from build123d import *

# Parameters (mm, degrees)
ESQUISSE1_R                  = 65
BOSS_EXTRU_1_DEPTH           = 8
ESQUISSE2_R                  = 63
ENL_V_MAT_EXTRU_1_DEPTH      = 6
BOSS_EXTRU_2_DEPTH           = 6
R_P_TITION_CIRCULAIRE1_COUNT = 8
COQUE1_DEPTH                 = 8
CHAMFER1_SIZE                = 3


# Read off the part's stored shape, not the designer's step: Coque1
with BuildPart() as part:
    # Esquisse1 → Boss.-Extru.1 (new body)
    with BuildSketch(Plane(origin=(0, 0, 0), x_dir=(1, 0, 0), z_dir=(0, 1, 0))):
        with Locations(Location((0, 0, 0), (0, 0, 270))):
            Circle(ESQUISSE1_R)
    extrude(amount=BOSS_EXTRU_1_DEPTH)

    # Esquisse2 → Enlèv. mat.-Extru.1 (cut)
    with BuildSketch(Plane(origin=(0, 8, 0), x_dir=(1, 0, 0), z_dir=(0, 1, 0))):
        with Locations(Location((0, 0, 0), (0, 0, 270))):
            Circle(ESQUISSE2_R)
    extrude(amount=-ENL_V_MAT_EXTRU_1_DEPTH, mode=Mode.SUBTRACT)

    # Esquisse3 → Boss.-Extru.2 (add)
    with BuildSketch(Plane(origin=(0, 2, 0), x_dir=(1, 0, 0), z_dir=(0, 1, 0))):
        with BuildLine():
            Line((-41.321316613, -33.189588629), (-17.610927668, -9.479199685))
            ThreePointArc((-17.610927668, -9.479199685), (-18.47759065, -7.653668647), (-19.155612754, -5.75))
            Line((-19.155612754, -5.75), (-52.687166369, -5.75))
            ThreePointArc((-52.687166369, -5.75), (-48.965615223, -20.282221915), (-41.321316613, -33.189588629))
        make_face()
        with BuildLine():
            Line((-36.942576794, -38.003236965), (-13.60185835, -14.662518522))
            ThreePointArc((-13.60185835, -14.662518522), (-14.142135624, -14.142135624), (-14.662518522, -13.60185835))
            Line((-14.662518522, -13.60185835), (-38.003236965, -36.942576794))
            ThreePointArc((-38.003236965, -36.942576794), (-37.476659403, -37.476659403), (-36.942576794, -38.003236965))
        make_face()
    boss_extru_2 = extrude(amount=BOSS_EXTRU_2_DEPTH)

    # Répétition circulaire1: Boss.-Extru.2 ×8 about axis
    r_p_tition_circulaire1_axis = Axis((0, 0, 0), (0, 1, 0))
    for i in range(1, R_P_TITION_CIRCULAIRE1_COUNT):
        add(boss_extru_2.rotate(r_p_tition_circulaire1_axis, i * 360 / R_P_TITION_CIRCULAIRE1_COUNT))

    # Coque1 outline → Coque1 (cut)
    with BuildSketch(Plane(origin=(0, 0, 0), x_dir=(1, 0, 0), z_dir=(0, 1, 0))):
        with BuildLine():
            Line((-50.407712704, 7.75), (-20.589742592, 7.75))
            ThreePointArc((-20.589742592, 7.75), (-20.325349715, 8.419035512), (-20.039224164, 9.079069055))
            Line((-20.039224164, 9.079069055), (-41.123713031, 30.163557923))
            ThreePointArc((-41.123713031, 30.163557923), (-47.117856158, 19.516855051), (-50.407712704, 7.75))
        make_face()
        with BuildLine():
            Line((20.589742592, 7.75), (50.407712704, 7.75))
            ThreePointArc((50.407712704, 7.75), (47.117856158, 19.516855051), (41.123713031, 30.163557923))
            Line((41.123713031, 30.163557923), (20.039224164, 9.079069055))
            ThreePointArc((20.039224164, 9.079069055), (20.325349715, 8.419035512), (20.589742592, 7.75))
        make_face()
        with BuildLine():
            ThreePointArc((-7.75, 50.407712704), (-19.516855051, 47.117856158), (-30.163557923, 41.123713031))
            Line((-30.163557923, 41.123713031), (-9.079069055, 20.039224164))
            ThreePointArc((-9.079069055, 20.039224164), (-8.419035512, 20.325349715), (-7.75, 20.589742592))
            Line((-7.75, 20.589742592), (-7.75, 50.407712704))
        make_face()
        with BuildLine():
            ThreePointArc((30.163557923, 41.123713031), (19.516855051, 47.117856158), (7.75, 50.407712704))
            Line((7.75, 50.407712704), (7.75, 20.589742592))
            ThreePointArc((7.75, 20.589742592), (8.419035512, 20.325349715), (9.079069055, 20.039224164))
            Line((9.079069055, 20.039224164), (30.163557923, 41.123713031))
        make_face()
        with BuildLine():
            ThreePointArc((41.123713031, -30.163557923), (47.117856158, -19.516855051), (50.407712704, -7.75))
            Line((50.407712704, -7.75), (20.589742592, -7.75))
            ThreePointArc((20.589742592, -7.75), (20.325349715, -8.419035512), (20.039224164, -9.079069055))
            Line((20.039224164, -9.079069055), (41.123713031, -30.163557923))
        make_face()
        with BuildLine():
            ThreePointArc((7.75, -50.407712704), (19.516855051, -47.117856158), (30.163557923, -41.123713031))
            Line((30.163557923, -41.123713031), (9.079069055, -20.039224164))
            ThreePointArc((9.079069055, -20.039224164), (8.419035512, -20.325349715), (7.75, -20.589742592))
            Line((7.75, -20.589742592), (7.75, -50.407712704))
        make_face()
        with BuildLine():
            ThreePointArc((-30.163557923, -41.123713031), (-19.516855051, -47.117856158), (-7.75, -50.407712704))
            Line((-7.75, -50.407712704), (-7.75, -20.589742592))
            ThreePointArc((-7.75, -20.589742592), (-8.419035512, -20.325349715), (-9.079069055, -20.039224164))
            Line((-9.079069055, -20.039224164), (-30.163557923, -41.123713031))
        make_face()
        with BuildLine():
            ThreePointArc((-50.407712704, -7.75), (-47.117856158, -19.516855051), (-41.123713031, -30.163557923))
            Line((-41.123713031, -30.163557923), (-20.039224164, -9.079069055))
            ThreePointArc((-20.039224164, -9.079069055), (-20.325349715, -8.419035512), (-20.589742592, -7.75))
            Line((-20.589742592, -7.75), (-50.407712704, -7.75))
        make_face()
    extrude(amount=COQUE1_DEPTH, mode=Mode.SUBTRACT)

    # Chamfer1
    chamfer1_edges = [part.edges().sort_by_distance(p)[0] for p in [
        (0, 2, -63),
    ]]
    chamfer(chamfer1_edges, length=CHAMFER1_SIZE)


solid = part.part
Verification items for the finished model (mm, model axes). A direction names the side the tool comes from. Give positions to 0.01 mm unless a question says otherwise; leave off trailing zeros.
1) Depth check by flat-ended pin: pin 1 Ø1.5 at (y, z) = (6.5, 50) entering from +X; pin 2 Ø4 at (x, y) = (29, 6) entering from -Z; pin 3 Ø4 at (x, y) = (-36, 2.5) entering from +Z. Enter the tip coordinate at first touch or a pass-through.
2) Draft check along Z on faces 4 (the cylindrical face through (20.477, 4.958, -48.885)), 5 (the flat face through (-25.44, 4.96, 26.5)), 6 (the flat face through (-26, 8, 26)). Enter one of: pulls with the +Z half, pulls with the -Z half, needs draft (parallel to the pull), parting line crosses it, or undercut.
3) Thickness scan on line 1 along X through (y, z) = (6.3, 0); line 2 along X through (y, z) = (6, -8); line 3 along Z through (x, y) = (38.5, 1.5). Record the ranges inside material, lowest first.
4) Set-up check for faces 1 (the flat face through (53.3, 8, -34)), 2 (the flat face through (-26.5, 4.96, -25.44)), 3 (the flat face through (-7.75, 4, -35)): record each of +Z, -Z, +X, -X, +Y, -Y from which the full face is reachable in a straight line by a thin tool's end or side.
5) Sectioned sample at A-A, the plane y = 3.5. Count the separate pieces of the cut face and the enclosed holes in it, then the cut area to 3 significant figures.
Answers:
1. pin 1: stops at x = 42.42
1. pin 2: stops at z = -59.13
1. pin 3: stops at z = 55.4
2. face 4: undercut
2. face 5: undercut
2. face 6: needs draft
3. line 1: x = -65 to -63, -53 to -20, 20 to 53, 63 to 65
3. line 2: x = -64.51 to -62.49, -52.39 to -50.37, -20.49 to -18.33, 18.33 to 20.49, 50.37 to 52.39, 62.49 to 64.51
3. line 3: z = -52.37 to -27.54, -7.75 to 7.75, 27.54 to 52.37
4. face 1: +Z, -Z, +X, -X, +Y
4. face 2: +Y
4. face 3: +Y, -Y
5. separate pieces: 17
5. enclosed holes: 9
5. area: 3,280 mm2
